```python
from build123d import *

# Parameters (mm, degrees)
BOSS_EXTRUDE1_DEPTH = 2.5
SKETCH3_W           = 7
SKETCH3_H           = 5
BOSS_EXTRUDE2_DEPTH = 135
SKETCH4_R           = 1.705
CUT_EXTRUDE1_DEPTH  = 5
LPATTERN1_COUNT     = 17
LPATTERN1_PITCH     = 5


with BuildPart() as part:
    # Sketch1 → Boss-Extrude1 (new body)
    with BuildSketch(Plane(origin=(0, 0, 0), x_dir=(1, 0, 0), z_dir=(0, 1, 0))):
        Polygon((4.210526316, 15), (-5.789473684, 15), (-5.789473684, 5), (-15.789473684, 5), (-15.789473684, -5), (-5.789473684, -5), (-5.789473684, -15), (4.210526316, -15), (4.210526316, -5), (14.210526316, -5), (14.210526316, 5), (4.210526316, 5), align=None)
    extrude(amount=-BOSS_EXTRUDE1_DEPTH)

    # Sketch3 → Boss-Extrude2 (add)
    with BuildSketch(Plane(origin=(0, 0, 0), x_dir=(1, 0, 0), z_dir=(0, 1, 0))):
        with Locations((-10.365258463, -0.095034863)):
            Rectangle(SKETCH3_W, SKETCH3_H)
        with Locations((8.634741537, -0.095034863)):
            Rectangle(SKETCH3_W, SKETCH3_H)
    extrude(amount=BOSS_EXTRUDE2_DEPTH)

    # Sketch4 → Cut-Extrude1 (cut, symmetric)
    with BuildSketch(Plane.XY):
        with Locations(Location((-10.0595209, 125, 0), (0, 0, 180))):
            Circle(SKETCH4_R)
        with Locations(Location((8.29517143, 125, 0), (0, 0, 180))):
            Circle(SKETCH4_R)
    cut_extrude1 = extrude(amount=CUT_EXTRUDE1_DEPTH, both=True, mode=Mode.SUBTRACT)

    # LPattern1: Cut-Extrude1 ×17
    with Locations(*[(0, -i * LPATTERN1_PITCH, 0) for i in range(1, LPATTERN1_COUNT)]):
        add(cut_extrude1, mode=Mode.SUBTRACT)


solid = part.part
```
Input: part model. Units: mm. Frame: model coordinates. A direction names the side the tool comes from. Give positions to 0.01 mm unless a question says otherwise; leave off trailing zeros. Write each loop counter-clockwise with the first axis right and the second up, starting at its lowest first coordinate (ties: lowest second). Pieces come first, ordered by that corner, then holes. Notation, with made-up numbers: (-16.5, -31.5) - (17.5, -31.5) arc R13 cw to (17.5, -16.5) - close; hole circle Ø6 at (-17, 77.5). An arc over 180 degrees is marked (long way). Write item = value, one per line. Start each with the question number.
1. Ray query, L1, parallel to X at y = 90, z = 0; L2, parallel to Y at x = -5.25, z = 13; L3, parallel to X at y = 104, z = 1.5. Return the intervals inside material, ascending.
2. Access query for faces 1 (the flat face through (4.211, -1, 10)), 2 (the flat face through (9, -1, -5)), 3 (the flat face through (5.135, 67, 0)), 4 (the flat face through (-11, 67, 2.595)). Directions: +Z, -Z, +X, -X, +Y, -Y. A direction counts if a zero-diameter tool reaches every point of the face in a straight line with its end or side. Return the directions, or none.
3. Mould query, pull axis X, two halves, no side actions, for faces 5 (the flat face through (14.211, -1, 0)), 6 (the cylindrical face through (7.38, 73.56, 0.13)), 7 (the flat face through (-11, 67, -2.405)). Classes: released by +X, released by -X, zero draft, split by the parting line, or undercut.
4. Section query B-B, the plane y = 85. Output: boundary loops of the cut face in (x, z), then the cut area to 3 significant figures.
5. First-contact query: pin 1 Ø3 at (x, y) = (8, -2) entering from +Z; pin 2 Ø3 at (x, y) = (-6, 97.5) entering from +Z; pin 3 Ø1.2 at (y, z) = (-1, 10.5) entering from +X; pin 4 Ø3 at (x, z) = (5, 3) entering from +Y. Flat tips, straight axial feed; report the tip coordinate or a pass-through.
6. Section query D-D, the plane x = -3.5. Output: boundary loops of the cut face in (y, z).
7. Section query C-C, the plane z = 9.75. Output: boundary loops of the cut face in (x, y).
8. Section query A-A, the plane y = 24. Output: boundary loops of the cut face in (x, z).
Check sheet entries:
q1.L1 = -13.87 to -11.76, -8.35 to -6.87, 5.13 to 6.59, 10 to 12.13
q1.L2 = -2.5 to 0
q1.L3 = -13.87 to -11.44, -8.68 to -6.87, 5.13 to 6.91, 9.68 to 12.13
q2.face_1 = +Z, +X, +Y, -Y
q2.face_2 = -Z, +X, +Y, -Y
q2.face_3 = +Z, -Z, +Y
q2.face_4 = +Z, +X, -X, +Y
q3.face_5 = released by +X
q3.face_6 = undercut
q3.face_7 = zero draft
q4.outline = (-13.87, -2.4) - (-11.76, -2.4) - (-11.76, 2.6) - (-13.87, 2.6) - close; (-8.35, -2.4) - (-6.87, -2.4) - (-6.87, 2.6) - (-8.35, 2.6) - close; (5.13, -2.4) - (6.59, -2.4) - (6.59, 2.6) - (5.13, 2.6) - close; (10, -2.4) - (12.13, -2.4) - (12.13, 2.6) - (10, 2.6) - close
q4.area = 35.9 mm2
q5.pin_1 = 5
q5.pin_2 = 2.6
q5.pin_3 = 4.21
q5.pin_4 = 135
q6.outline = (-2.5, -15) - (0, -15) - (0, 15) - (-2.5, 15) - close
q7.outline = (-5.79, -2.5) - (4.21, -2.5) - (4.21, 0) - (-5.79, 0) - close
q8.outline = (-13.87, -2.4) - (-6.87, -2.4) - (-6.87, 2.6) - (-13.87, 2.6) - close; (5.13, -2.4) - (12.13, -2.4) - (12.13, 2.6) - (5.13, 2.6) - close
